Answer from the drawing. Dimensions are ordinates in mm from the lowest x, y and z of the part. A direction names the side the tool comes from. Give positions to 0.01 mm unless a question says otherwise; leave off trailing zeros. Order: outer loops, then holes, each group sorted by start corner. A loop starts at its lowest first (then second) coordinate and runs counter-clockwise, first axis right, second up. Notation, with made-up numbers: M 87.25,70.5 L 97.25,70.5 A22 ccw 97.25,103.5 Z; hole C -13.5,26.25 d10. An arc over 180 degrees is marked long. One line per item, written item: value.
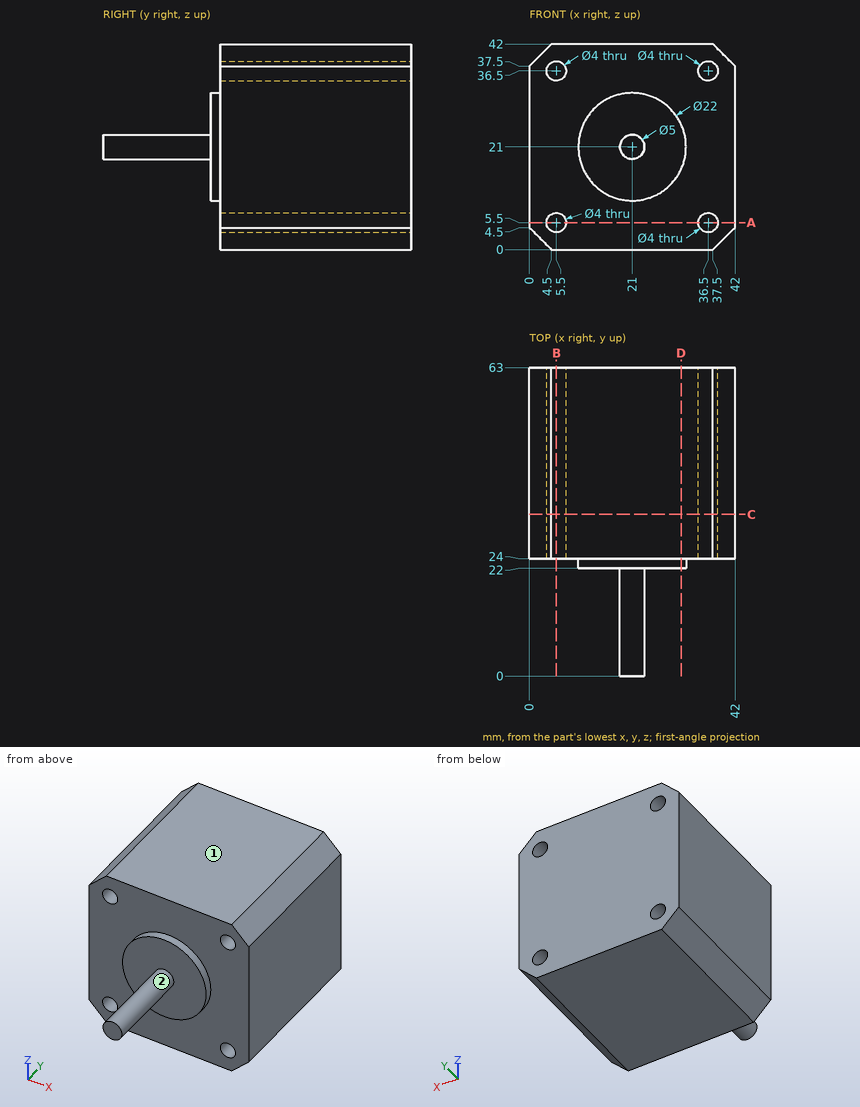
(1) Find the intervals of material crossed by probe 1 along Z at (x, y) = (36.5, 46.5); probe 2 along X at (y, z) = (50, 36), in increasing order. Write a range as from..to.
Findings:
probe 1: z = 0..3.5, 7.5..34.5, 38.5..42
probe 2: x = 0..3.56, 7.44..34.56, 38.44..42
(2) Section B-B, the plane x = 5.5 is taken. Give the vertices of the cut face in (y, z).
Findings:
outline: M 24,0 L 63,0 L 63,3.5 L 24,3.5 Z; M 24,7.5 L 63,7.5 L 63,34.5 L 24,34.5 Z; M 24,38.5 L 63,38.5 L 63,42 L 24,42 Z
(3) Section C-C, the plane y = 33 is taken. Give the vertices of the cut face in (x, z), then the cut area to 3 significant figures.
Findings:
outline: M 0,4.5 L 4.5,0 L 37.5,0 L 42,4.5 L 42,37.5 L 37.5,42 L 4.5,42 L 0,37.5 Z; hole C 5.5,5.5 d4; hole C 5.5,36.5 d4; hole C 36.5,5.5 d4; hole C 36.5,36.5 d4
area: 1,670 mm^2
(4) Section D-D, the plane x = 31 is taken. Give the vertices of the cut face in (y, z).
Findings:
outline: M 22,16.42 L 24,16.42 L 24,0 L 63,0 L 63,42 L 24,42 L 24,25.58 L 22,25.58 Z
(5) Given P1, Ø6.5, axis at x = 36.5, z = 5.5, coming from the -Y side; P2, Ø4.5, axis at x = 5.5, z = 5.5, coming from the +Y side, each flat-ended and moving along its own axis, determine where each tip first touches the part or whether it passes through.
Findings:
P1: stops at y = 24
P2: stops at y = 63
(6) Which of the six approach directions +Z, -Z, +X, -X, +Y, -Y give full straight-line access (tool end or side, diameter ignored) to the marked faces 1 and 2?
Findings:
face 1: +Z, +X, -X, +Y, -Y
face 2: -Y
(7) Section A-A, the plane z = 5.5 is taken. Give the vertices of the cut face in (x, y), then the cut area to 3 significant figures.
Findings:
outline: M 0,24 L 3.5,24 L 3.5,63 L 0,63 Z; M 7.5,24 L 34.5,24 L 34.5,63 L 7.5,63 Z; M 38.5,24 L 42,24 L 42,63 L 38.5,63 Z
area: 1,330 mm^2
